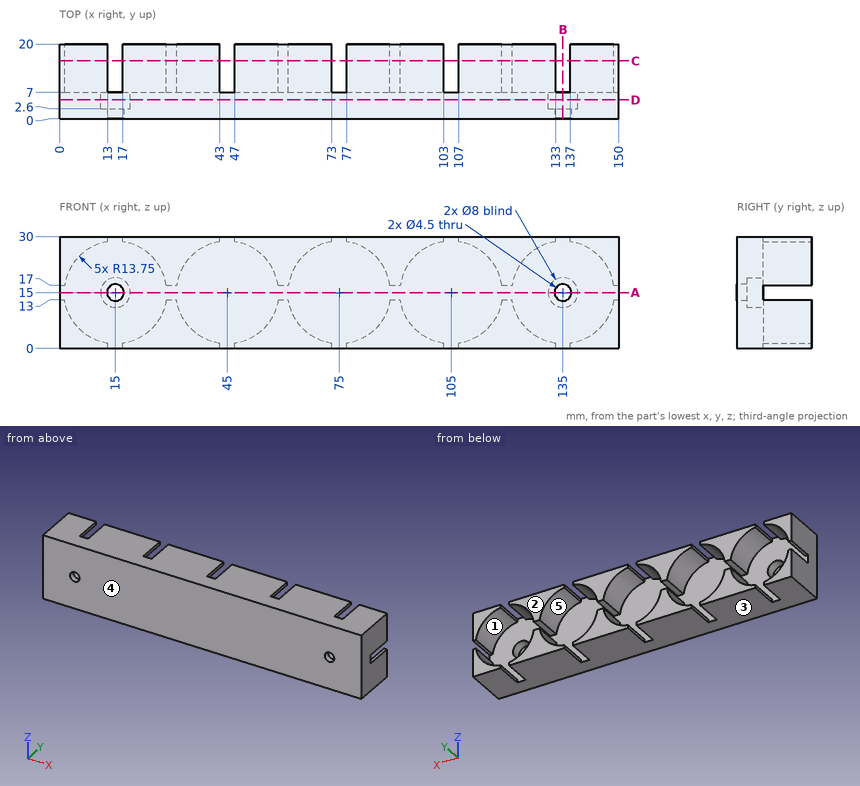
Source: three-view drawing plus pictorial views. Frame: mm from the lowest corner of the part. A direction names the side the tool comes from. Coordinates: 2 decimals unless noted, no trailing zeros. Write each loop counter-clockwise with the first axis right and the second up, starting at its lowest first coordinate (ties: lowest second). Pieces come first, ordered by that corner, then holes. Notation, with made-up numbers: (48.5, 69) -> (98.5, 69) arc R28 cw to (98.5, 105) -> close; hole circle Ø1 at (65.5, 5). An arc over 180 degrees is marked (long way). Answer as a JSON object with one key per item and string values.
1. Section B-B on x = 135. Return the cut outline in (y, z), then the cut area to 3 significant figures.
Result set:
{"outline": "(0, 0) -> (7, 0) -> (7, 11) -> (2.6, 11) -> (2.6, 12.75) -> (0, 12.75) -> close; (0, 17.25) -> (2.6, 17.25) -> (2.6, 19) -> (7, 19) -> (7, 30) -> (0, 30) -> close", "area": "163 mm2"}
2. Material intervals for line 1 (Z direction, x = 15, y = 1.35); line 2 (X direction, y = 7.75, z = 20.25); line 3 (Z direction, x = 135, y = 6.05), sorted ascending. Write a range as from..to.
Result set:
{"line 1": "z = 0..12.75, 17.25..30", "line 2": "x = 0..2.29, 27.71..32.29, 57.71..62.29, 87.71..92.29, 117.71..122.29, 147.71..150", "line 3": "z = 0..11, 19..30"}
3. Section A-A on z = 15. Return the cut outline in (x, y).
Result set:
{"outline": "(0, 0) -> (12.75, 0) -> (12.75, 2.6) -> (11, 2.6) -> (11, 7) -> (0, 7) -> close; (17.25, 0) -> (132.75, 0) -> (132.75, 2.6) -> (131, 2.6) -> (131, 7) -> (19, 7) -> (19, 2.6) -> (17.25, 2.6) -> close; (137.25, 0) -> (150, 0) -> (150, 7) -> (139, 7) -> (139, 2.6) -> (137.25, 2.6) -> close"}
4. Section C-C on y = 15.5. Count the separate pieces of the cut face and the enclosed holes in it, then the cut area to 3 significant figures.
Result set:
{"separate pieces": "12", "enclosed holes": "0", "area": "1,430 mm2"}
5. First-contact query: P1, Ø10, axis at y = 3, z = 13.5, coming from the -X side; P2, Ø6.5, axis at x = 15, z = 13, coming from the +Y side. Flat tips, straight axial feed; report the tip coordinate or a pass-through.
Result set:
{"P1": "stops at x = 0", "P2": "stops at y = 7"}
6. Section D-D on y = 5. Return the cut outline in (x, z), then the cut area to 3 significant figures.
Result set:
{"outline": "(0, 0) -> (150, 0) -> (150, 30) -> (0, 30) -> close; hole circle Ø8 at (15, 15); hole circle Ø8 at (135, 15)", "area": "4,400 mm2"}
7. Access query for the marked faces 4 and 5. Directions: +Z, -Z, +X, -X, +Y, -Y. A direction counts if a zero-diameter tool reaches every point of the face in a straight line with its end or side. Return the directions, or none.
Result set:
{"face 4": "+Z, -Z, +X, -X, -Y", "face 5": "+Y"}
8. Mould query, pull axis Z, two halves, no side actions, for the marked faces 1, 2 and 3. Classes: released by +Z, released by -Z, zero draft, split by the parting line, or undercut.
Result set:
{"face 1": "undercut", "face 2": "zero draft", "face 3": "released by -Z"}
